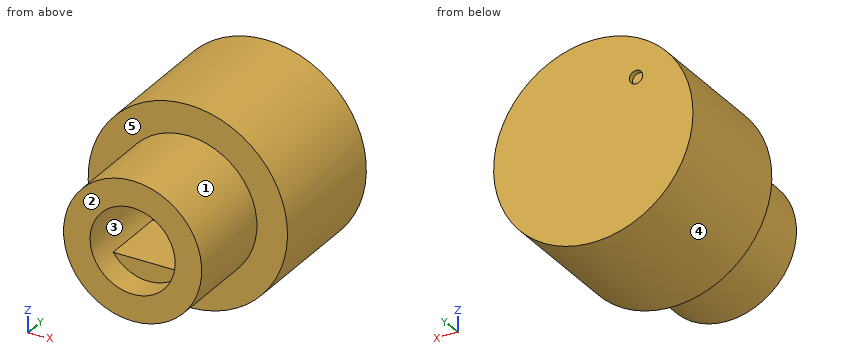
from build123d import *

# Parameters (mm, degrees)
SKETCH1_R           = 5.2
SKETCH1_R_2         = 3.2
BOSS_EXTRUDE1_DEPTH = 7
SKETCH2_R           = 7.5
BOSS_EXTRUDE2_DEPTH = 10
BOSS_EXTRUDE3_START = 1
BOSS_EXTRUDE3_DEPTH = 1
BOSS_EXTRUDE4_START = 5
BOSS_EXTRUDE4_DEPTH = 5
SKETCH5_R           = 0.5
CUT_EXTRUDE1_DEPTH  = 0.4


with BuildPart() as part:
    # Sketch1 → Boss-Extrude1 (new body)
    with BuildSketch(Plane(origin=(0, 0, 0), x_dir=(1, 0, 0), z_dir=(0, 1, 0))):
        with Locations(Location((0, 0, 0), (0, 0, 270))):
            Circle(SKETCH1_R)
        with Locations(Location((0, 0, 0), (0, 0, 270))):
            Circle(SKETCH1_R_2, mode=Mode.SUBTRACT)
    extrude(amount=BOSS_EXTRUDE1_DEPTH)

    # Sketch2 → Boss-Extrude2 (add)
    with BuildSketch(Plane(origin=(0, 7, 0), x_dir=(1, 0, 0), z_dir=(0, 1, 0))):
        with Locations(Location((0, 0, 0), (0, 0, 270))):
            Circle(SKETCH2_R)
    extrude(amount=BOSS_EXTRUDE2_DEPTH)

    # Sketch3 → Boss-Extrude3 (add)
    with BuildSketch(Plane.XZ.offset(-7).offset(BOSS_EXTRUDE3_START)):
        with BuildLine():
            Line((3.174901573, 0.4), (-3.174901573, 0.4))
            ThreePointArc((-3.174901573, 0.4), (-3.19371923, 0.20039332), (-3.2, 0))
            ThreePointArc((-3.2, 0), (-3.19371923, -0.20039332), (-3.174901573, -0.4))
            Line((-3.174901573, -0.4), (3.174901573, -0.4))
            ThreePointArc((3.174901573, -0.4), (3.19371923, -0.20039332), (3.2, 0))
            ThreePointArc((3.2, 0), (3.19371923, 0.20039332), (3.174901573, 0.4))
        make_face()
    extrude(amount=-BOSS_EXTRUDE3_DEPTH)

    # Sketch4 → Boss-Extrude4 (add)
    with BuildSketch(Plane.XZ.offset(-7).offset(BOSS_EXTRUDE4_START)):
        with BuildLine():
            Line((2.645751311, -1.8), (-2.645751311, -1.8))
            ThreePointArc((-2.645751311, -1.8), (0, -3.2), (2.645751311, -1.8))
        make_face()
    extrude(amount=-BOSS_EXTRUDE4_DEPTH)

    # Sketch5 → Cut-Extrude1 (cut)
    with BuildSketch(Plane(origin=(0, 17, 0), x_dir=(1, 0, 0), z_dir=(0, 1, 0))):
        with Locations(Location((-3.213938048, -3.830222216, 0), (0, 0, 270))):
            Circle(SKETCH5_R)
    extrude(amount=-CUT_EXTRUDE1_DEPTH, mode=Mode.SUBTRACT)


solid = part.part
Could you check a few things on this model? Use its own coordinates, in mm. Face numbers are marked on the shaded views. A direction names the side the tool comes from. Give positions to 0.01 mm unless a question says otherwise; leave off trailing zeros. Order: outer loops, then holes, each group sorted by start corner. A loop starts at its lowest first (then second) coordinate and runs counter-clockwise, first axis right, second up. Notation, with made-up numbers: (79, -28.75) - (109, -28.75) arc R7 ccw to (109, -23.75) - close; hole circle Ø10 at (31.5, 48.5). An arc over 180 degrees is marked (long way). One line per question, with ' | ' between items. Start each with the question number.
Item 1: I need wall thicknesses on probe 1 along X at (y, z) = (2.75, 0); probe 2 along Y at (x, z) = (5, -2.5); probe 3 along X at (y, z) = (11.75, 0.25). Which ranges of each line are inside material? Lowest first, please. Write a range as [from, to].
Item 2: I want a section at A-A on y = 6.5. Write out the boundary of the cut face in (x, z).
Item 3: For the marked faces 1 and 2, which set-ups out of +Z, -Z, +X, -X, +Y, -Y let a thin tool reach every point of the face, with its end or its side?
Item 4: I want a section at D-D on y = 3. Write out the boundary of the cut face in (x, z), then the cut area to 3 significant figures.
Item 5: Thinking about a two-plate mould opening in X: for the marked faces 3, 4 and 5, which applies, pulls with the +X half, pulls with the -X half, needs draft (parallel to the pull), parting line crosses it, or undercut?
Item 6: I'm going to push flat-ended pins straight in: pin 1 Ø0.7 at (x, z) = (0, -1) entering from -Y; pin 2 Ø1.5 at (x, y) = (2, 5.5) entering from +Z; pin 3 Ø1.1 at (x, y) = (1.5, 6.5) entering from +Z; pin 4 Ø1 at (y, z) = (3.5, -6) entering from +X. Where does each tip first touch, or does it pass through?
Item 7: I want a section at C-C on z = 0. Write out the boundary of the cut face in (x, y), then the cut area to 3 significant figures.
Item 8: I want a section at B-B on x = 0. Write out the boundary of the cut face in (y, z).
Verdict:
1) probe 1: [-5.2, -3.2], [3.2, 5.2] | probe 2: [7, 17] | probe 3: [-7.5, 7.5]
2) outline: circle Ø10.4 at (0, 0); hole (-3.17, -0.4) arc R3.2 ccw to (-2.65, -1.8) - (2.65, -1.8) arc R3.2 ccw to (3.17, -0.4) - close; hole (-3.17, 0.4) - (3.17, 0.4) arc R3.2 ccw to start
3) face 1: -Y | face 2: +Z, -Z, +X, -X, -Y
4) outline: circle Ø10.4 at (0, 0); hole (-2.65, -1.8) - (2.65, -1.8) arc R3.2 ccw (long way) to start | area: 58.0 mm^2
5) face 3: undercut | face 4: parting line crosses it | face 5: needs draft
6) pin 1: y = 7 | pin 2: z = 5.05 | pin 3: z = 7.39 | pin 4: through
7) outline: (-7.5, 7) - (-5.2, 7) - (-5.2, 0) - (-3.2, 0) - (-3.2, 6) - (3.2, 6) - (3.2, 0) - (5.2, 0) - (5.2, 7) - (7.5, 7) - (7.5, 17) - (-7.5, 17) - close | area: 184 mm^2
8) outline: (0, -5.2) - (7, -5.2) - (7, -7.5) - (17, -7.5) - (17, 7.5) - (7, 7.5) - (7, 5.2) - (0, 5.2) - (0, 3.2) - (7, 3.2) - (7, 0.4) - (6, 0.4) - (6, -0.4) - (7, -0.4) - (7, -1.8) - (2, -1.8) - (2, -3.2) - (0, -3.2) - close
